```python
from build123d import *

# Parameters (mm, degrees)
BOSS_EXTRUDE1_DEPTH   = 6
M2X0_4_TAPPED_HOLE1_D = 1.6
FILLET1_R             = 2.54


with BuildPart() as part:
    # Sketch1 → Boss-Extrude1 (new body)
    with BuildSketch(Plane.XY):
        with BuildLine():
            Line((-31.4941, 0), (-26.4941, 0))
            Line((-26.4941, 0), (-26.4941, 1.524))
            ThreePointArc((-26.4941, 1.524), (-25.750151224, 3.320051224), (-23.9541, 4.064))
            Line((-23.9541, 4.064), (23.9541, 4.064))
            ThreePointArc((23.9541, 4.064), (25.750151224, 3.320051224), (26.4941, 1.524))
            Line((26.4941, 1.524), (26.4941, 0))
            Line((26.4941, 0), (31.4941, 0))
            Line((31.4941, 0), (31.4941, 10.156063356))
            Line((31.4941, 10.156063356), (17.963402264, 10.156063356))
            Line((17.963402264, 10.156063356), (17.963402264, 8.886063356))
            ThreePointArc((17.963402264, 8.886063356), (18.668015075, 8.290353704), (18.034, 7.62))
            Line((18.034, 7.62), (-18.034, 7.62))
            ThreePointArc((-18.034, 7.62), (-18.668015075, 8.290353704), (-17.963402264, 8.886063356))
            Line((-17.963402264, 8.886063356), (-17.963402264, 10.156063356))
            Line((-17.963402264, 10.156063356), (-31.4941, 10.156063356))
            Line((-31.4941, 10.156063356), (-31.4941, 0))
        make_face()
    extrude(amount=BOSS_EXTRUDE1_DEPTH)

    # M2x0.4 Tapped Hole1 (through all)
    with Locations(Plane(origin=(0, 0, 0), x_dir=(-1, 0, 0), z_dir=(0, -1, 0))):
        with Locations((28.9941, -3), (-28.9941, -3)):
            Hole(M2X0_4_TAPPED_HOLE1_D / 2)

    # Fillet1
    # the kernel refuses this fillet: 2.54 mm, written as the material it takes off along each edge
    with BuildSketch(Plane(origin=(-26.4941, -6.35, 0), x_dir=(-1, 0, 0), z_dir=(0, 1, 0)), Plane(origin=(26.4941, 1.524, 0), x_dir=(1, 0, 0), z_dir=(0, -1, 0))) as fillet1_piece_1:
        with BuildLine():
            CenterArc((FILLET1_R, FILLET1_R), FILLET1_R, 180, 90)
            Line((0, FILLET1_R), (0, 0))
            Line((0, 0), (FILLET1_R, 0))
        make_face()
    extrude(amount=7.874, mode=Mode.SUBTRACT)
    with BuildSketch(Plane(origin=(-23.9541, 1.524, 0), x_dir=(-1, 0, 0), z_dir=(0, -1, 0))) as fillet1_piece_2:
        with BuildLine():
            CenterArc((2.54 + FILLET1_R, -FILLET1_R), FILLET1_R, 90, 90)
            Line((2.54, -FILLET1_R), (2.54, 0))
            Line((2.54, 0), (2.54 + FILLET1_R, 0))
        make_face()
    revolve(axis=Axis((-23.9541, 1.524, 0), (0, 0, -1)), revolution_arc=90, mode=Mode.SUBTRACT)
    with BuildSketch(Plane(origin=(23.9541, 1.524, 0), x_dir=(0, 1, 0), z_dir=(-1, 0, 0))) as fillet1_piece_3:
        with BuildLine():
            CenterArc((2.54 + FILLET1_R, -FILLET1_R), FILLET1_R, 90, 90)
            Line((2.54, -FILLET1_R), (2.54, 0))
            Line((2.54, 0), (2.54 + FILLET1_R, 0))
        make_face()
    revolve(axis=Axis((23.9541, 1.524, 0), (0, 0, -1)), revolution_arc=90, mode=Mode.SUBTRACT)
    with BuildSketch(Plane(origin=(-26.4941, -6.35, 6), x_dir=(-1, 0, 0), z_dir=(0, 1, 0)), Plane(origin=(26.4941, 1.524, 6), x_dir=(1, 0, 0), z_dir=(0, -1, 0))) as fillet1_piece_4:
        with BuildLine():
            CenterArc((FILLET1_R, -FILLET1_R), FILLET1_R, 90, 90)
            Line((0, -FILLET1_R), (0, 0))
            Line((0, 0), (FILLET1_R, 0))
        make_face()
    extrude(amount=7.874, mode=Mode.SUBTRACT)
    with BuildSketch(Plane(origin=(-23.9541, 1.524, 6), x_dir=(-1, 0, 0), z_dir=(0, -1, 0))) as fillet1_piece_5:
        with BuildLine():
            CenterArc((2.54 + FILLET1_R, FILLET1_R), FILLET1_R, 180, 90)
            Line((2.54, FILLET1_R), (2.54, 0))
            Line((2.54, 0), (2.54 + FILLET1_R, 0))
        make_face()
    revolve(axis=Axis((-23.9541, 1.524, 6), (0, 0, -1)), revolution_arc=90, mode=Mode.SUBTRACT)
    with BuildSketch(Plane(origin=(-23.9541, 4.064, 6), x_dir=(0, 1, 0), z_dir=(1, 0, 0))) as fillet1_piece_6:
        with BuildLine():
            CenterArc((FILLET1_R, -FILLET1_R), FILLET1_R, 90, 90)
            Line((0, -FILLET1_R), (0, 0))
            Line((0, 0), (FILLET1_R, 0))
        make_face()
    extrude(amount=47.9082, mode=Mode.SUBTRACT)
    with BuildSketch(Plane(origin=(23.9541, 1.524, 6), x_dir=(0, 1, 0), z_dir=(-1, 0, 0))) as fillet1_piece_7:
        with BuildLine():
            CenterArc((2.54 + FILLET1_R, FILLET1_R), FILLET1_R, 180, 90)
            Line((2.54, FILLET1_R), (2.54, 0))
            Line((2.54, 0), (2.54 + FILLET1_R, 0))
        make_face()
    revolve(axis=Axis((23.9541, 1.524, 6), (0, 0, -1)), revolution_arc=90, mode=Mode.SUBTRACT)
    with BuildSketch(Plane(origin=(-31.4941, 16.506063356, 0), x_dir=(1, 0, 0), z_dir=(0, -1, 0)), Plane(origin=(31.4941, -6.35, 0), x_dir=(-1, 0, 0), z_dir=(0, 1, 0))) as fillet1_piece_8:
        with BuildLine():
            CenterArc((FILLET1_R, FILLET1_R), FILLET1_R, 180, 90)
            Line((0, FILLET1_R), (0, 0))
            Line((0, 0), (FILLET1_R, 0))
        make_face()
    extrude(amount=22.856063356, mode=Mode.SUBTRACT)
    with BuildSketch(Plane(origin=(-31.4941, 16.506063356, 6), x_dir=(1, 0, 0), z_dir=(0, -1, 0)), Plane(origin=(31.4941, -6.35, 6), x_dir=(-1, 0, 0), z_dir=(0, 1, 0))) as fillet1_piece_9:
        with BuildLine():
            CenterArc((FILLET1_R, -FILLET1_R), FILLET1_R, 90, 90)
            Line((0, -FILLET1_R), (0, 0))
            Line((0, 0), (FILLET1_R, 0))
        make_face()
    extrude(amount=22.856063356, mode=Mode.SUBTRACT)
    with BuildSketch(Plane(origin=(-23.9541, 4.064, 0), x_dir=(0, 1, 0), z_dir=(1, 0, 0))) as fillet1_piece_10:
        with BuildLine():
            CenterArc((FILLET1_R, FILLET1_R), FILLET1_R, 180, 90)
            Line((0, FILLET1_R), (0, 0))
            Line((0, 0), (FILLET1_R, 0))
        make_face()
    extrude(amount=47.9082, mode=Mode.SUBTRACT)
    with BuildSketch(Plane(origin=(31.4941, 10.156063356, -6.35), x_dir=(0, -1, 0), z_dir=(0, 0, 1)), Plane(origin=(-31.4941, 10.156063356, -6.35), x_dir=(1, 0, 0), z_dir=(0, 0, 1))) as fillet1_piece_11:
        with BuildLine():
            CenterArc((FILLET1_R, -FILLET1_R), FILLET1_R, 90, 90)
            Line((0, -FILLET1_R), (0, 0))
            Line((0, 0), (FILLET1_R, 0))
        make_face()
    extrude(amount=18.7, mode=Mode.SUBTRACT)


solid = part.part
```
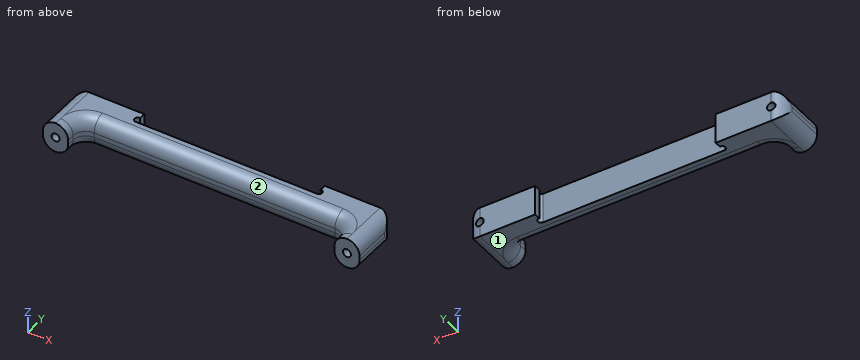
Verification items for the finished model (mm, model axes). Face numbers are marked on the shaded views. A direction names the side the tool comes from. Coordinates: 2 decimals unless noted, no trailing zeros. Write each loop counter-clockwise with the first axis right and the second up, starting at its lowest first coordinate (ties: lowest second). Pieces come first, ordered by that corner, then holes. Notation, with made-up numbers: M 36,4.25 L 91,4.25 A15 ccw 91,24.25 Z; hole C -29,-3 d6. An arc over 180 degrees is marked long. One line per item, written item: value.
Item 1: Section check B-B, the plane y = 3.5. State how many separate pieces and enclosed holes the cut face has, plus the area to 3 significant figures.
Check sheet entries:
separate pieces: 2
enclosed holes: 2
area: 54.3 mm^2
Item 2: Scan lines: line 1 along X through (y, z) = (6.5, 3); line 2 along X through (y, z) = (8.25, 3); line 3 along X through (y, z) = (9.25, 2.75). Record each from-to range of solid material in increasing order.
Check sheet entries:
line 1: x = -31.49 to -29.79, -28.19 to 28.19, 29.79 to 31.49
line 2: x = -31.41 to -29.79, -28.19 to -18.67, 18.67 to 28.19, 29.79 to 31.41
line 3: x = -30.9 to -29.75, -28.23 to -17.96, 17.96 to 28.23, 29.75 to 30.9
Item 3: Section check C-C, the plane x = 20. Record the boundary of the cut face in (y, z), plus the area to 3 significant figures.
Check sheet entries:
outline: M 4.06,2.54 A2.54 ccw 6.6,0 L 10.16,0 L 10.16,6 L 6.6,6 A2.54 ccw 4.06,3.46 Z
area: 33.8 mm^2
Item 4: Section check A-A, the plane x = -3. Record the boundary of the cut face in (y, z), plus the area to 3 significant figures.
Check sheet entries:
outline: M 4.06,2.54 A2.54 ccw 6.6,0 L 7.62,0 L 7.62,6 L 6.6,6 A2.54 ccw 4.06,3.46 Z
area: 18.6 mm^2
Item 5: Access from +Z, -Z, +X, -X, +Y, -Y to the whole of each face (thin tool, end or side, straight path). Record for the marked faces 1 and 2.
Check sheet entries:
face 1: -Z, +X, -X, +Y, -Y
face 2: +Z, -Y
Item 6: Gauge pin test, flat ends, axial feed: pin 1 Ø1.4 at (y, z) = (9, 2.5) entering from +X; pin 2 Ø3 at (x, z) = (14, 1.5) entering from -Y. Record the tip position at first contact, or that the pin passes through.
Check sheet entries:
pin 1: stops at x = 31.4
pin 2: stops at y = 4.06
